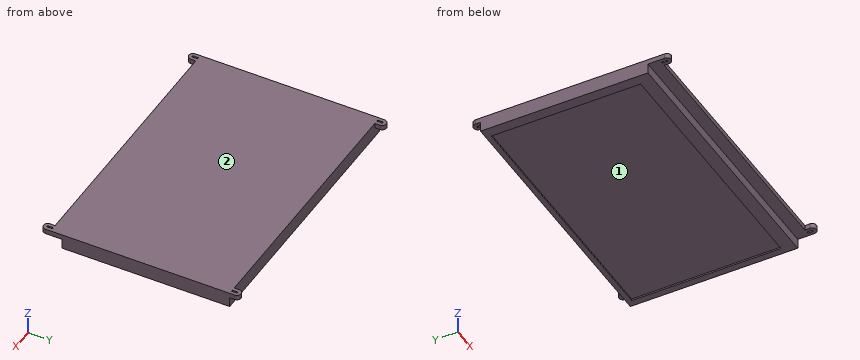
```python
from build123d import *

# Parameters (mm, degrees)
ESBO_O1_W                = 164
ESBO_O1_H                = 107
RESSALTO_EXTRUS_O1_DEPTH = 4.5
EXTRUS_O_FINA2_DEPTH     = 3
ESBO_O3_W                = 164
ESBO_O3_H                = 7
CORTE_EXTRUS_O1_DEPTH    = 6
ESBO_O5_W                = 153.790549152
ESBO_O5_H                = 89.226156431
CORTE_EXTRUS_O2_DEPTH    = 1


with BuildPart() as part:
    # Esboço1 → Ressalto-extrusão1 (new, symmetric)
    with BuildSketch(Plane.XY):
        with Locations((-7.64158605, 1.401746725)):
            Rectangle(ESBO_O1_W, ESBO_O1_H)
    extrude(amount=RESSALTO_EXTRUS_O1_DEPTH, both=True)

    # Esboço2 → Extrusão-Fina2 (add)
    with BuildSketch(Plane.XY.offset(4.5)):
        with BuildLine():
            Line((-89.64158605, 54.901746725), (-89.64158605, 57.901746725))
            ThreePointArc((-89.64158605, 57.901746725), (-87.14158605, 60.401746725), (-84.64158605, 57.901746725))
            Line((-84.64158605, 57.901746725), (-84.64158605, 54.901746725))
            Line((-84.64158605, 54.901746725), (-86.64158605, 54.901746725))
            Line((-86.64158605, 54.901746725), (-86.64158605, 57.901746725))
            ThreePointArc((-86.64158605, 57.901746725), (-87.14158605, 58.401746725), (-87.64158605, 57.901746725))
            Line((-87.64158605, 57.901746725), (-87.64158605, 54.901746725))
            Line((-87.64158605, 54.901746725), (-89.64158605, 54.901746725))
        make_face()
        with BuildLine():
            Line((69.35841395, 54.901746725), (69.35841395, 57.901746725))
            ThreePointArc((69.35841395, 57.901746725), (71.85841395, 60.401746725), (74.35841395, 57.901746725))
            Line((74.35841395, 57.901746725), (74.35841395, 54.901746725))
            Line((74.35841395, 54.901746725), (72.35841395, 54.901746725))
            Line((72.35841395, 54.901746725), (72.35841395, 57.901746725))
            ThreePointArc((72.35841395, 57.901746725), (71.85841395, 58.401746725), (71.35841395, 57.901746725))
            Line((71.35841395, 57.901746725), (71.35841395, 54.901746725))
            Line((71.35841395, 54.901746725), (69.35841395, 54.901746725))
        make_face()
        with BuildLine():
            Line((-84.64158605, -52.098253275), (-84.64158605, -55.098253275))
            ThreePointArc((-84.64158605, -55.098253275), (-87.14158605, -57.598253275), (-89.64158605, -55.098253275))
            Line((-89.64158605, -55.098253275), (-89.64158605, -52.098253275))
            Line((-89.64158605, -52.098253275), (-87.64158605, -52.098253275))
            Line((-87.64158605, -52.098253275), (-87.64158605, -55.098253275))
            ThreePointArc((-87.64158605, -55.098253275), (-87.14158605, -55.598253275), (-86.64158605, -55.098253275))
            Line((-86.64158605, -55.098253275), (-86.64158605, -52.098253275))
            Line((-86.64158605, -52.098253275), (-84.64158605, -52.098253275))
        make_face()
        with BuildLine():
            Line((74.35841395, -52.098253275), (74.35841395, -55.098253275))
            ThreePointArc((74.35841395, -55.098253275), (71.85841395, -57.598253275), (69.35841395, -55.098253275))
            Line((69.35841395, -55.098253275), (69.35841395, -52.098253275))
            Line((69.35841395, -52.098253275), (71.35841395, -52.098253275))
            Line((71.35841395, -52.098253275), (71.35841395, -55.098253275))
            ThreePointArc((71.35841395, -55.098253275), (71.85841395, -55.598253275), (72.35841395, -55.098253275))
            Line((72.35841395, -55.098253275), (72.35841395, -52.098253275))
            Line((72.35841395, -52.098253275), (74.35841395, -52.098253275))
        make_face()
    extrude(amount=-EXTRUS_O_FINA2_DEPTH)

    # Esboço3 → Corte-extrusão1 (cut)
    with BuildSketch(Plane(origin=(0, 0, -4.5), x_dir=(-1, 0, 0), z_dir=(0, 0, -1))):
        with Locations((7.64158605, -48.598253275)):
            Rectangle(ESBO_O3_W, ESBO_O3_H)
    extrude(amount=-CORTE_EXTRUS_O1_DEPTH, mode=Mode.SUBTRACT)

    # Esboço5 → Corte-extrusão2 (cut)
    with BuildSketch(Plane(origin=(0, 0, -4.5), x_dir=(-1, 0, 0), z_dir=(0, 0, -1))):
        with Locations((6.536860626, 7.288668509)):
            Rectangle(ESBO_O5_W, ESBO_O5_H)
    extrude(amount=-CORTE_EXTRUS_O2_DEPTH, mode=Mode.SUBTRACT)


solid = part.part
```
Work out the finished part from the listing and answer in its coordinate system (mm). Face numbers are marked on the shaded views. Give positions to 0.01 mm unless a question says otherwise; leave off trailing zeros. Write each loop counter-clockwise with the first axis right and the second up, starting at its lowest first coordinate (ties: lowest second). Pieces come first, ordered by that corner, then holes. Notation, with made-up numbers: (53.25, -29.75) -> (76.25, -29.75) arc R14 cw to (76.25, -23.75) -> close; hole circle Ø4 at (50.25, 73.25). An arc over 180 degrees is marked (long way). Write item = value, one per line.
Q1. Section C-C on z = -1 is taken. Determine the outline of the cut face in (x, y).
Computed values:
outline = (-89.64, -45.1) -> (74.36, -45.1) -> (74.36, 54.9) -> (-89.64, 54.9) -> close
Q2. Flat-ended cylindrical pins translate along their axes: pin 1 Ø10 at (x, y) = (-47, -48.5) entering from -Z; pin 2 Ø1.5 at (x, y) = (3, -36.5) entering from -Z; pin 3 Ø0.5 at (x, z) = (25.5, -4) entering from -Y; pin 4 Ø1.5 at (x, z) = (-41, 3.5) entering from -Y. Find the tip coordinate at first contact, or state that the pin passes through.
Computed values:
pin_1 = -4.5
pin_2 = -3.5
pin_3 = -45.1
pin_4 = -52.1
Q3. For a pull along X with two mould halves and no side action, classify the marked faces 1 and 2 as pulls with the +X half, pulls with the -X half, needs draft (parallel to the pull), parting line crosses it, or undercut.
Computed values:
face_1 = undercut
face_2 = needs draft
Q4. Section B-B on y = -26 is taken. Determine the outline of the cut face in (x, z), and give its area (3 significant figures).
Computed values:
outline = (-89.64, -4.5) -> (-83.43, -4.5) -> (-83.43, -3.5) -> (70.36, -3.5) -> (70.36, -4.5) -> (74.36, -4.5) -> (74.36, 4.5) -> (-89.64, 4.5) -> close
area = 1,320 mm^2
Q5. Section A-A on x = -29 is taken. Determine the outline of the cut face in (y, z).
Computed values:
outline = (-52.1, 1.5) -> (-45.1, 1.5) -> (-45.1, -4.5) -> (-37.32, -4.5) -> (-37.32, -3.5) -> (51.9, -3.5) -> (51.9, -4.5) -> (54.9, -4.5) -> (54.9, 4.5) -> (-52.1, 4.5) -> close
Q6. Consider line 1 along Z through (x, y) = (-28, -35); line 2 along Y through (x, z) = (45, -2.75); line 3 along Y through (x, z) = (27, 4). Determine where each line is inside the solid, lowest interval first.
Computed values:
line_1 = -3.5 to 4.5
line_2 = -45.1 to 54.9
line_3 = -52.1 to 54.9
